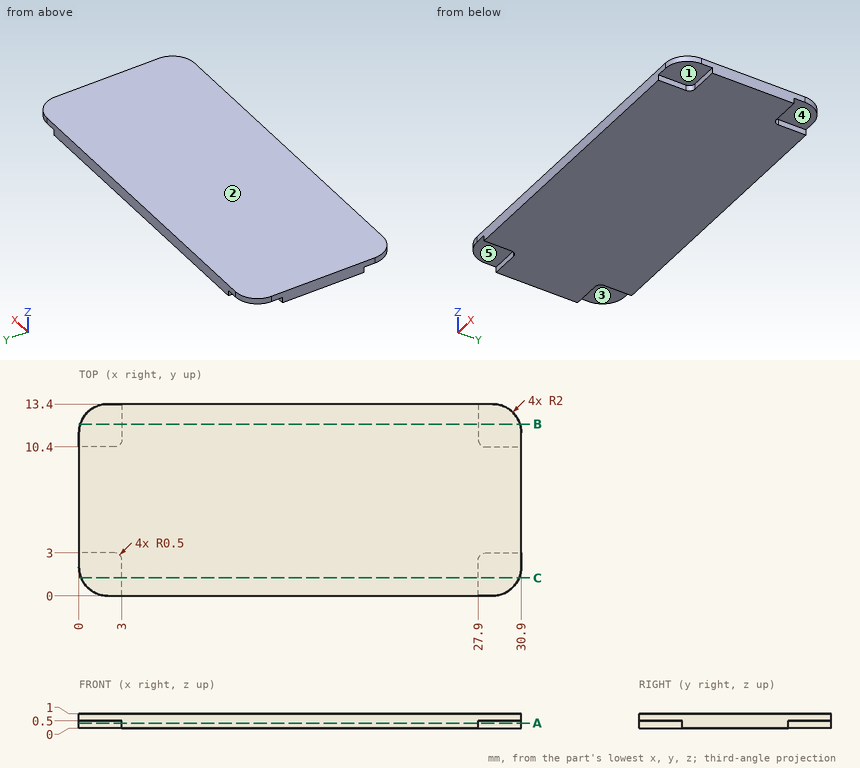
Study the drawing (mm; zero at the part's minimum x, y, z) and answer. A direction names the side the tool comes from. Give positions to 0.01 mm unless a question says otherwise; leave off trailing zeros. Loops run counter-clockwise (first coordinate to the right, second up) from the corner with the lowest first, then second, coordinate; pieces in that order, holes last. Notation, with made-up numbers: (4.5, -12) -> (42.5, -12) arc R17 cw to (42.5, 20) -> close; hole circle Ø5 at (-24, 64.5). An arc over 180 degrees is marked (long way). Write item = value, one per line. Start each with the question number.
(1) Find section B-B on y = 12. Give the vertices of the cut face in (x, z), and give its area (3 significant figures).
(2) Find section C-C on y = 1.25. Give the vertices of the cut face in (x, z), and give its area (3 significant figures).
(3) Given pin 1 Ø0.6 at (y, z) = (12.5, 0) entering from -X; pin 2 Ø3.5 at (x, y) = (1.5, 1.5) entering from -Z; pin 3 Ø2.5 at (x, y) = (30, 1) entering from -Z; pin 4 Ø0.6 at (x, z) = (1, 0.5) entering from +Y, each flat-ended and moving along its own axis, determine where each tip first touches the part or whether it passes through.
(4) Find section A-A on z = 0.35. Give the vertices of the cut face in (x, y).
(5) Which of the six approach directions +Z, -Z, +X, -X, +Y, -Y give full straight-line access (tool end or side, diameter ignored) to the marked faces 1, 2, 3, 4 and 5?
(6) Find the intervals of material crossed by probe 1 along X at (y, z) = (11.5, 0.95); probe 2 along X at (y, z) = (2, 0.2); probe 3 along Z at (x, y) = (2, 2.5), in increasing order. Write a range as from..to.
From the geometry:
q1.outline = (0.09, 0.5) -> (3, 0.5) -> (3, 0) -> (27.9, 0) -> (27.9, 0.5) -> (30.81, 0.5) -> (30.81, 1) -> (0.09, 1) -> close
q1.area = 27.8 mm^2
q2.outline = (0.15, 0.5) -> (3, 0.5) -> (3, 0) -> (27.9, 0) -> (27.9, 0.5) -> (30.75, 0.5) -> (30.75, 1) -> (0.15, 1) -> close
q2.area = 27.8 mm^2
q3.pin_1 = 3
q3.pin_2 = 0
q3.pin_3 = 0.5
q3.pin_4 = 13.27
q4.outline = (0, 3) -> (2.5, 3) arc R0.5 cw to (3, 2.5) -> (3, 0) -> (27.9, 0) -> (27.9, 2.5) arc R0.5 cw to (28.4, 3) -> (30.9, 3) -> (30.9, 10.4) -> (28.4, 10.4) arc R0.5 cw to (27.9, 10.9) -> (27.9, 13.4) -> (3, 13.4) -> (3, 10.9) arc R0.5 cw to (2.5, 10.4) -> (0, 10.4) -> close
q5.face_1 = -Z, +X, -Y
q5.face_2 = +Z, +X, -X, +Y, -Y
q5.face_3 = -Z, -X, +Y
q5.face_4 = -Z, +X, +Y
q5.face_5 = -Z, -X, -Y
q6.probe_1 = 0..30.9
q6.probe_2 = 3..27.9
q6.probe_3 = 0.5..1
